from build123d import *

# Parameters (mm, degrees)
SKETCH1_R           = 9.5
BOSS_EXTRUDE1_DEPTH = 25
SKETCH2_R           = 5
CUT_EXTRUDE1_DEPTH  = 20
SKETCH3_R           = 2
CUT_EXTRUDE2_DEPTH  = 29.381331893


with BuildPart() as part:
    # Sketch1 → Boss-Extrude1 (new body)
    with BuildSketch(Plane(origin=(0, 0, 0), x_dir=(1, 0, 0), z_dir=(0, 1, 0))):
        with Locations(Location((0, 0, 0), (0, 0, 270))):
            Circle(SKETCH1_R)
    extrude(amount=BOSS_EXTRUDE1_DEPTH)

    # Sketch2 → Cut-Extrude1 (cut)
    with BuildSketch(Plane(origin=(0, 25, 0), x_dir=(1, 0, 0), z_dir=(0, 1, 0))):
        with Locations(Location((0, 0, 0), (0, 0, 270))):
            Circle(SKETCH2_R)
    extrude(amount=-CUT_EXTRUDE1_DEPTH, mode=Mode.SUBTRACT)

    # Sketch3 → Cut-Extrude2 (cut, through all)
    with BuildSketch(Plane.XZ):
        with Locations(Location((0, 0, 0), (0, 0, 270))):
            Circle(SKETCH3_R)
    extrude(amount=-CUT_EXTRUDE2_DEPTH, mode=Mode.SUBTRACT)


solid = part.part
CAD build for the part. Positions are in the model's coordinates, mm. A direction names the side the tool comes from. Coordinates: 2 decimals unless noted, no trailing zeros. Write each loop counter-clockwise with the first axis right and the second up, starting at its lowest first coordinate (ties: lowest second). Pieces come first, ordered by that corner, then holes. Notation, with made-up numbers: (-18.5, 64) - (37.5, 64) arc R14 cw to (37.5, 77) - close; hole circle Ø8 at (65, 8). An arc over 180 degrees is marked (long way). Use a Markdown table: item, result. Add a question column.
Item 1: Mould opens along Z. For faces 3 (the face through (-4.88, 15.14, -1.08)), 4 (the face through (-4, 25, 4)), 5 (the face through (-5.78, 12.32, -7.54)) say: pulls with the +Z half, pulls with the -Z half, needs draft (parallel to the pull), parting line crosses it, or undercut.
Item 2: Band-saw the part on B-B, the plane x = 0. Give the cut face in (y, z).
Item 3: Band-saw the part on D-D, the plane z = -4. Give the cut face in (x, y).
Item 4: Band-saw the part on A-A, the plane z = 0. Give the cut face in (x, y).
Item 5: 3-axis set-ups, long thin cutter, end or side, ignore diameter. For faces 1 (the face through (0.1, 5, 2.2)), 2 (the face through (-2, 2, 0)): which of +Z, -Z, +X, -X, +Y, -Y reach the whole face in a straight line?
Item 6: Drill centre lines: L1, parallel to X at y = 20.5, z = 0; L2, parallel to X at y = 1.15, z = 0; L3, parallel to Y at x = -2.5, z = 2.25. Where is each one in solid material? Low to high. Write a range as from..to.
Item 7: Flat gauge pins, fed straight in: pin 1 (10 mm diameter, centred on x = -7.5, y = 8, fed in from -Z); pin 2 (8 mm diameter, centred on y = 10.5, z = 4.5, fed in from -X); pin 3 (2 mm diameter, centred on x = -6, y = 4, fed in from -Z). Where does each tip first touch, or does it go through?
Item 8: Band-saw the part on C-C, the plane y = 6. Give the cut face in (x, z).
Numbers:
| question | item | result |
|---|---|---|
| 1 | face 3 | undercut |
| 1 | face 4 | needs draft |
| 1 | face 5 | parting line crosses it |
| 2 | outline | (0, -9.5) - (25, -9.5) - (25, -5) - (5, -5) - (5, -2) - (0, -2) - close; (0, 2) - (5, 2) - (5, 5) - (25, 5) - (25, 9.5) - (0, 9.5) - close |
| 3 | outline | (-8.62, 0) - (8.62, 0) - (8.62, 25) - (3, 25) - (3, 5) - (-3, 5) - (-3, 25) - (-8.62, 25) - close |
| 4 | outline | (-9.5, 0) - (-2, 0) - (-2, 5) - (-5, 5) - (-5, 25) - (-9.5, 25) - close; (2, 0) - (9.5, 0) - (9.5, 25) - (5, 25) - (5, 5) - (2, 5) - close |
| 5 | face 1 | +Y |
| 5 | face 2 | +Y, -Y |
| 6 | L1 | -9.5..-5, 5..9.5 |
| 6 | L2 | -9.5..-2, 2..9.5 |
| 6 | L3 | 0..5 |
| 7 | pin 1 | z = -9.17 |
| 7 | pin 2 | x = -9.49 |
| 7 | pin 3 | z = -8.08 |
| 8 | outline | circle Ø19 at (0, 0); hole circle Ø10 at (0, 0) |
